The model under review builds one solid part; all positions refer to its coordinate system, in mm. A direction names the side the tool comes from. Round coordinates to 2 decimals unless told otherwise and drop trailing zeros. Write each loop counter-clockwise with the first axis right and the second up, starting at its lowest first coordinate (ties: lowest second). Pieces come first, ordered by that corner, then holes. Notation, with made-up numbers: (-2.75, 79) - (25.25, 79) arc R25 ccw to (25.25, 117) - close; hole circle Ø11 at (15, 82.5). An arc over 180 degrees is marked (long way). Return JSON: item names as keys, results as strings.
from build123d import *

# Parameters (mm, degrees)
F0_R     = 1.85
F1_DEPTH = 0.95
F2_W     = 4.5
F2_H     = 4.2
F3_DEPTH = 3.25
F4_R     = 2.09999
F5_R     = 1.15
F6_DEPTH = 25


# Not quite as in the source:
# - a fillet or chamfer is up to 0.001 mm smaller than in the source, because OpenCascade refuses the exact size


with BuildPart() as f1:
    # F0 (on Top) → F1 (new body)
    with BuildSketch(Plane.XY):
        with BuildLine():
            Line((9.5515289224, 0.7), (14.9, 0.7))
            Line((14.9, 0.7), (14.9, 4.9))
            Line((14.9, 4.9), (10.4, 4.9))
            Line((10.4, 4.9), (9.5515289224, 4.9))
            ThreePointArc((9.5515289224, 4.9), (9.4002214052, 4.9040911969), (9.2493560516, 4.916352832))
            Line((9.2493560516, 4.916352832), (3.1021728708, 5.583647168))
            ThreePointArc((3.1021728708, 5.583647168), (2.9513075171, 5.5959088031), (2.8, 5.6))
            ThreePointArc((2.8, 5.6), (0.8201010127, 4.7798989873), (0, 2.8))
            ThreePointArc((0, 2.8), (0.8201010127, 0.8201010127), (2.8, 0))
            ThreePointArc((2.8, 0), (2.9513075171, 0.0040911969), (3.1021728708, 0.016352832))
            Line((3.1021728708, 0.016352832), (9.2493560516, 0.683647168))
            ThreePointArc((9.2493560516, 0.683647168), (9.4002214052, 0.6959088031), (9.5515289224, 0.7))
        make_face()
        with Locations((2.8, 2.8)):
            Circle(F0_R, mode=Mode.SUBTRACT)
    extrude(amount=F1_DEPTH)

    # F2 (on face) → F3 (join)
    with BuildSketch(Plane.XY.offset(0.95)):
        with Locations((12.65, 2.8)):
            Rectangle(F2_W, F2_H)
    extrude(amount=F3_DEPTH)

    # F4 (radius 2.1 in the source; OpenCascade refuses exactly that, so slightly less here)
    f4_edges = [f1.edges().sort_by_distance(p)[0] for p in [
        (12.65, 4.9, 4.2),
        (12.65, 0.7, 4.2),
    ]]
    fillet(f4_edges, radius=F4_R)

    # F5 (on face) → F6 (cut)
    with BuildSketch(Plane.YZ.offset(14.9)):
        with Locations((2.8, 2.1)):
            Circle(F5_R)
    extrude(amount=-F6_DEPTH, mode=Mode.SUBTRACT)


solid = f1.part
(1) Add section A-A (z = 0.7). Write out the cut boundary in (x, y), plus the area to 3 significant figures.
Filled in:
{"outline": "(3.1, 0.02) - (9.25, 0.68) arc R2.8 cw to (9.55, 0.7) - (14.9, 0.7) - (14.9, 4.9) - (9.55, 4.9) arc R2.8 cw to (9.25, 4.92) - (3.1, 5.58) arc R2.8 ccw (long way) to start; hole circle Ø3.7 at (2.8, 2.8)", "area": "57.1 mm2"}
(2) Add section D-D (y = 3.55). Write out the cut boundary in (x, z), plus the area to 3 significant figures.
Filled in:
{"outline": "(0.1, 0) - (1.11, 0) - (1.11, 0.95) - (0.1, 0.95) - close; (4.49, 0) - (14.9, 0) - (14.9, 1.23) - (10.4, 1.23) - (10.4, 0.95) - (4.49, 0.95) - close; (10.4, 2.97) - (14.9, 2.97) - (14.9, 4.06) - (10.4, 4.06) - close", "area": "17.0 mm2"}
(3) Add section C-C (x = 3.25). Write out the cut boundary in (y, z), plus the area to 3 significant figures.
Filled in:
{"outline": "(0.03, 0) - (1.01, 0) - (1.01, 0.95) - (0.03, 0.95) - close; (4.59, 0) - (5.57, 0) - (5.57, 0.95) - (4.59, 0.95) - close", "area": "1.85 mm2"}
(4) Clearance check with flat-ended pins moving along their axes: pin 1 Ø1.5 at (x, z) = (8.5, 2) entering from -Y; pin 2 Ø1.1 at (x, z) = (12.5, 1) entering from -Y; pin 3 Ø2.5 at (y, z) = (3.5, 3) entering from -X; pin 4 Ø0.6 at (x, z) = (11.5, 1) entering from +Y. State where each tip first meets the part, or that it passes through.
Filled in:
{"pin 1": "passes through", "pin 2": "stops at y = 0.7", "pin 3": "stops at x = 10.4", "pin 4": "stops at y = 4.9"}
(5) For faces 4 (the flat face through (12, 0.7, 1)), 5 (the flat face through (6, 3, 0.95)), 6 (the flat face through (12, 4.9, 1)), list the 3-axis set-ups (+Z, -Z, +X, -X, +Y, -Y) from which the entire face can be reached by the end or side of a thin tool; tool diameter is ignored.
Filled in:
{"face 4": "+Z, -Z, +X, -Y", "face 5": "+Z, -X, +Y, -Y", "face 6": "+Z, -Z, +X, +Y"}
(6) Mouldability with a two-part tool opening along Y and no side actions: class faces 1 (the flat face through (10.4, 4, 3)), 2 (the cylindrical face through (12.68, 3.42, 3.07)), 3 (the flat face through (6.133, 0.345, 0.468)) as released by +Y, released by -Y, zero draft, split by the parting line, or undercut.
Filled in:
{"face 1": "zero draft", "face 2": "undercut", "face 3": "released by -Y"}
(7) Wall thickness on line 1 (Y direction, x = 13.15, z = 2.1); line 2 (Z direction, x = 12.55, y = 2.8); line 3 (Y direction, x = 2.8, z = 0.6): over which ranges is each line inside the solid? List them lowest first.
Filled in:
{"line 1": "y = 0.7 to 1.65, 3.95 to 4.9", "line 2": "z = 0 to 0.95, 3.25 to 4.2", "line 3": "y = 0 to 0.95, 4.65 to 5.6"}
